Design review of the part shown in the three views and the two pictorial views. Dimensions are in mm from the part's minimum x, y and z. A direction names the side the tool comes from. Coordinates: 2 decimals unless noted, no trailing zeros. Loops run counter-clockwise (first coordinate to the right, second up) from the corner with the lowest first, then second, coordinate; pieces in that order, holes last.
Q1. Add section C-C on z = 13.35. Give the boundary of the cut face in (x, y), and give its area (3 significant figures).
Q2. Add section A-A on z = 8. Give the boundary of the cut face in (x, y), and give its area (3 significant figures).
Q3. Add section B-B on x = 13.35. Give the boundary of the cut face in (y, z), and give its area (3 significant figures).
Q4. Wall thickness on probe 1 along Z at (x, y) = (21, 3.5); probe 2 along X at (y, z) = (0.8, 19.35) (3 decimals); probe 3 along Y at (x, z) = (12.5, 20.75): over which ranges is each line inside the solid? List them lowest first.
Q5. For P1, Ø3, axis at x = 19.35, z = 19.35, coming from the -Y side; P2, Ø3, axis at x = 20.5, z = 19, coming from the +Y side; P3, Ø5, axis at x = 8, z = 7.5, coming from the +Y side; P4, Ø1.5, axis at y = 4.5, z = 12.5, coming from the +X side, all flat-tipped, find the tip position at first contact; note any pin that passes through.
Q6. Machinability: for the marked faces 4 and 5, which of the approach directions +Z, -Z, +X, -X, +Y, -Y give a long, thin tool a straight path to every point of the face, cutting with its end or side? Answer none if there is none.
Q7. Add section D-D on x = 7.35. Give the boundary of the cut face in (y, z) (3 decimals), and give its area (3 significant figures).
Q8. Draft analysis for pull direction Z (two halves, no side actions). For the marked faces 1, 2 and 3, state which applies: released by +Z, released by -Z, zero draft, split by the parting line, or undercut.
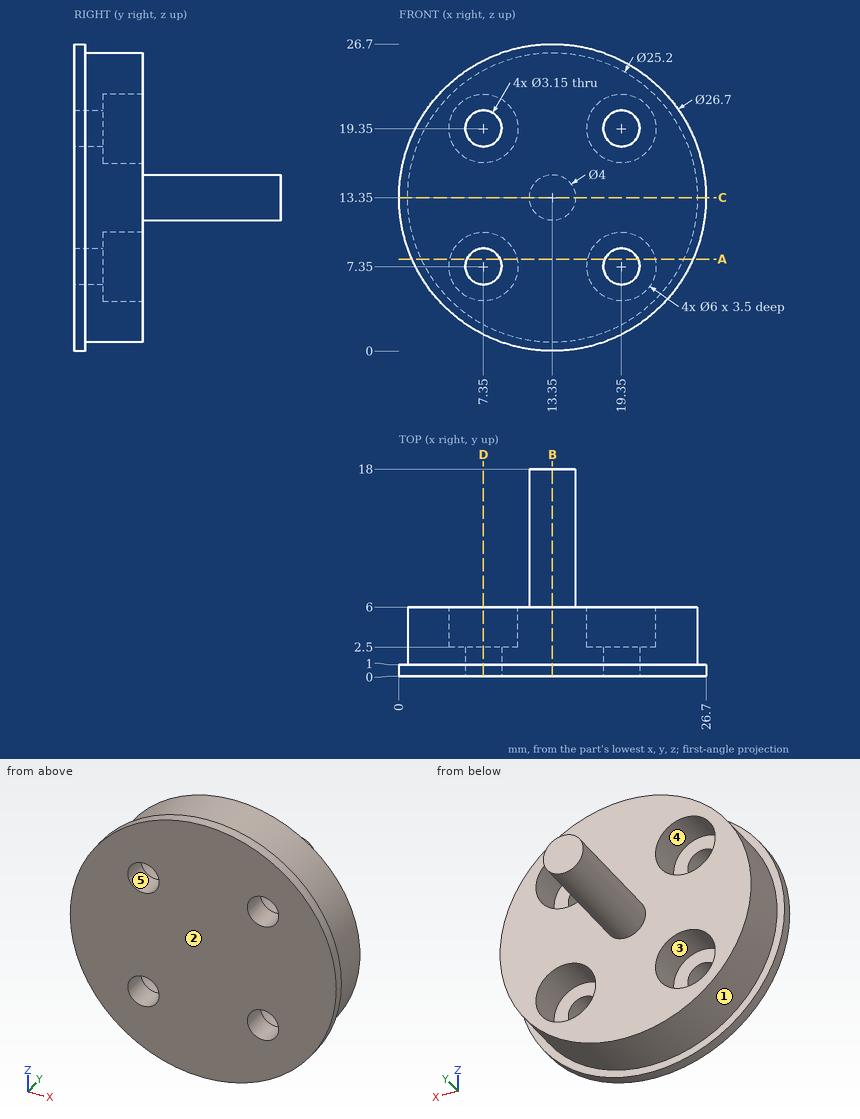
Entries:
1. outline: (0, 0) - (26.7, 0) - (26.7, 1) - (25.95, 1) - (25.95, 6) - (15.35, 6) - (15.35, 18) - (11.35, 18) - (11.35, 6) - (0.75, 6) - (0.75, 1) - (0, 1) - close
1. area: 201 mm2
2. outline: (1.12, 0) - (5.92, 0) - (5.92, 2.5) - (4.42, 2.5) - (4.42, 6) - (1.94, 6) - (1.94, 1) - (1.12, 1) - close; (8.78, 0) - (17.92, 0) - (17.92, 2.5) - (16.42, 2.5) - (16.42, 6) - (10.28, 6) - (10.28, 2.5) - (8.78, 2.5) - close; (20.78, 0) - (25.58, 0) - (25.58, 1) - (24.76, 1) - (24.76, 6) - (22.28, 6) - (22.28, 2.5) - (20.78, 2.5) - close
2. area: 83.2 mm2
3. outline: (0, 0) - (1, 0) - (1, 0.75) - (6, 0.75) - (6, 11.35) - (18, 11.35) - (18, 15.35) - (6, 15.35) - (6, 25.95) - (1, 25.95) - (1, 26.7) - (0, 26.7) - close
3. area: 201 mm2
4. probe 1: z = 3.34 to 4.84, 9.86 to 16.84, 21.86 to 23.36
4. probe 2: x = 1.424 to 5.775, 8.925 to 17.775, 20.925 to 25.276
4. probe 3: y = 0 to 6
5. P1: passes through
5. P2: stops at y = 2.5
5. P3: stops at y = 6
5. P4: stops at x = 25.95
6. face 4: +Y
6. face 5: +Y, -Y
7. outline: (0, 1.424) - (1, 1.424) - (1, 2.27) - (6, 2.27) - (6, 4.35) - (2.5, 4.35) - (2.5, 5.775) - (0, 5.775) - close; (0, 8.925) - (2.5, 8.925) - (2.5, 10.35) - (6, 10.35) - (6, 16.35) - (2.5, 16.35) - (2.5, 17.775) - (0, 17.775) - close; (0, 20.925) - (2.5, 20.925) - (2.5, 22.35) - (6, 22.35) - (6, 24.43) - (1, 24.43) - (1, 25.276) - (0, 25.276) - close
7. area: 76.9 mm2
8. face 1: split by the parting line
8. face 2: zero draft
8. face 3: undercut
